Build history of the part. All positions in model axes, mm. A direction names the side the tool comes from. Give positions to 0.01 mm unless a question says otherwise; leave off trailing zeros. Write each loop counter-clockwise with the first axis right and the second up, starting at its lowest first coordinate (ties: lowest second). Pieces come first, ordered by that corner, then holes. Notation, with made-up numbers: (79, 60) -> (94, 60) arc R30 ccw to (94, 89) -> close; hole circle Ø7 at (60, 13.25). An arc over 180 degrees is marked (long way). Put each result on its own line as item: value. Start each with the question number.
Item 1: Slice it at C-C, the plane y = 2. List the corners of the cut face in (x, z).
Item 2: Slice it at A-A, the plane z = 25. List the corners of the cut face in (x, y), plus the area to 3 significant figures.
Item 3: Flat gauge pin, fed straight in: pin 1 Ø10 at (x, y) = (-29, -4) entering from -Z. Where does the tip first touch, or does it go through?
Item 4: Slice it at B-B, the plane z = 45. List the corners of the cut face in (x, y), plus the area to 3 significant figures.
Item 5: Drill centre lines: line 1 along X through (y, z) = (3, 24); line 2 along X through (y, z) = (12, 25); line 3 along X through (y, z) = (-17, 41). Where is each one in solid material? Low to high.
Item 6: Tool access for faces 5 (the flat face through (38, -20, 36)), 6 (the flat face through (74.234, 0, 25)), 7 (the flat face through (-2, 0, 0)): list every direction of +Z, -Z, +X, -X, +Y, -Y with a clear straight run to the whole face (end or side of a thin tool).
Item 7: Two-plate mould, pull along Y, no slides. Class faces 1 (the flat face through (-2, -25, 25)), 2 (the flat face through (-2, 25, 25)), 3 (the cylindrical face through (63.877, -0.28, 28.252)), 4 (the flat face through (-150, 0, 25)): pulls with the +Y half, pulls with the -Y half, needs draft (parallel to the pull), parting line crosses it, or undercut.
```python
from build123d import *

# Parameters (mm, degrees)
SKETCH1_W               = 300
SKETCH1_H               = 50
BOSS_EXTRUDE1_DEPTH     = 50
CUT_EXTRUDE1_DEPTH      = 166.831239518
CUT_EXTRUDE1_DEPTH_BACK = 166.831239518
SKETCH2_R               = 15
CUT_EXTRUDE2_START      = -5
SKETCH3_W               = 50
SKETCH3_H               = 50
CUT_EXTRUDE2_DEPTH      = 40
BOSS_EXTRUDE2_REACH     = 166.393
SKETCH4_R               = 15


with BuildPart() as part:
    # Sketch1 → Boss-Extrude1 (new body)
    with BuildSketch(Plane.XY):
        Rectangle(SKETCH1_W, SKETCH1_H)
    extrude(amount=BOSS_EXTRUDE1_DEPTH)

    # Sketch2 → Cut-Extrude1 (cut, two sides: drawn at the far end of the back side and taken through both)
    with BuildSketch(Plane(origin=(0, 25, 0), x_dir=(1, 0, 0), z_dir=(0, 1, 0)).offset(-CUT_EXTRUDE1_DEPTH_BACK)):
        with Locations(Location((-126.266078419, -25, 0), (0, 0, 270))):
            Circle(SKETCH2_R)
    extrude(amount=CUT_EXTRUDE1_DEPTH + CUT_EXTRUDE1_DEPTH_BACK, mode=Mode.SUBTRACT)

    # Sketch3 → Cut-Extrude2 (cut)
    with BuildSketch(Plane(origin=(0, 25, 0), x_dir=(1, 0, 0), z_dir=(0, 1, 0)).offset(CUT_EXTRUDE2_START)):
        with Locations((49.233921581, -25)):
            Rectangle(SKETCH3_W, SKETCH3_H)
    extrude(amount=-CUT_EXTRUDE2_DEPTH, mode=Mode.SUBTRACT)

    # Sketch4 → Boss-Extrude2 (add, up to next)
    with BuildSketch(Plane(origin=(0, -20, 0), x_dir=(1, 0, 0), z_dir=(0, 1, 0)), mode=Mode.PRIVATE) as boss_extrude2_sk1:
        with Locations(Location((49.233921581, -25, 0), (0, 0, 90))):
            Circle(SKETCH4_R)
    boss_extrude2_tool1 = extrude(boss_extrude2_sk1.sketch, amount=BOSS_EXTRUDE2_REACH, mode=Mode.PRIVATE) - part.part
    add(boss_extrude2_tool1.solids().sort_by_distance((49.233922, -20, 25))[0])


solid = part.part
```
Values follow:
1. outline: (-150, 0) -> (24.23, 0) -> (24.23, 50) -> (-150, 50) -> close; circle Ø30 at (49.23, 25); (74.23, 0) -> (150, 0) -> (150, 50) -> (74.23, 50) -> close; hole circle Ø30 at (-126.27, 25)
2. outline: (-150, -25) -> (-141.27, -25) -> (-141.27, 25) -> (-150, 25) -> close; (-111.27, -25) -> (150, -25) -> (150, 25) -> (-111.27, 25) -> close; hole (24.23, -20) -> (34.23, -20) -> (34.23, 20) -> (24.23, 20) -> close; hole (64.23, -20) -> (74.23, -20) -> (74.23, 20) -> (64.23, 20) -> close
2. area: 12,700 mm2
3. pin 1: z = 0
4. outline: (-150, -25) -> (150, -25) -> (150, 25) -> (-150, 25) -> close; hole (24.23, -20) -> (74.23, -20) -> (74.23, 20) -> (24.23, 20) -> close
4. area: 13,000 mm2
5. line 1: -150 to -141.23, -111.3 to 24.23, 34.27 to 64.2, 74.23 to 150
5. line 2: -150 to -141.27, -111.27 to 24.23, 34.23 to 64.23, 74.23 to 150
5. line 3: -150 to 24.23, 74.23 to 150
6. face 5: none
6. face 6: +Z, -Z
6. face 7: -Z, +X, -X, +Y, -Y
7. face 1: pulls with the -Y half
7. face 2: pulls with the +Y half
7. face 3: undercut
7. face 4: needs draft
